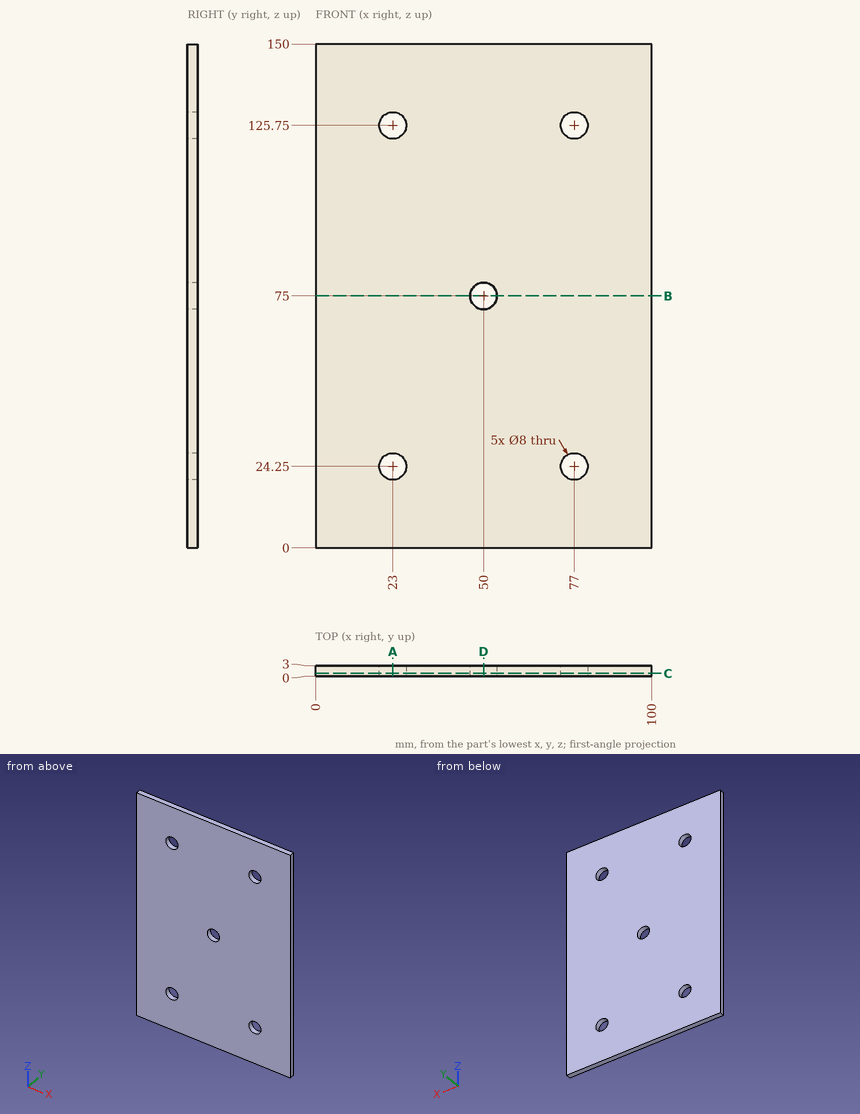
Answer from the drawing. Dimensions are ordinates in mm from the lowest x, y and z of the part. Coordinates: 2 decimals unless noted, no trailing zeros. Loops run counter-clockwise (first coordinate to the right, second up) from the corner with the lowest first, then second, coordinate; pieces in that order, holes last. Notation, with made-up numbers: (48, -34.75) -> (81, -34.75) arc R26 ccw to (81, -1.75) -> close; hole circle Ø6 at (23, -0.5). An arc over 180 degrees is marked (long way). Return JSON: item names as keys, results as strings.
Item 1: Find section D-D (x = 50). Determine the outline of the cut face in (y, z).
Answers:
{"outline": "(0, 0) -> (3, 0) -> (3, 71) -> (0, 71) -> close; (0, 79) -> (3, 79) -> (3, 150) -> (0, 150) -> close"}
Item 2: Find section A-A (x = 23). Determine the outline of the cut face in (y, z).
Answers:
{"outline": "(0, 0) -> (3, 0) -> (3, 20.25) -> (0, 20.25) -> close; (0, 28.25) -> (3, 28.25) -> (3, 121.75) -> (0, 121.75) -> close; (0, 129.75) -> (3, 129.75) -> (3, 150) -> (0, 150) -> close"}
Item 3: Find the intervals of material crossed by probe 1 along Z at (x, y) = (77, 1.8); probe 2 along X at (y, z) = (1.35, 126); probe 3 along X at (y, z) = (1.4, 21.5), in increasing order.
Answers:
{"probe 1": "z = 0 to 20.25, 28.25 to 121.75, 129.75 to 150", "probe 2": "x = 0 to 19.01, 26.99 to 73.01, 80.99 to 100", "probe 3": "x = 0 to 20.1, 25.9 to 74.1, 79.9 to 100"}
Item 4: Find section B-B (z = 75). Determine the outline of the cut face in (x, y).
Answers:
{"outline": "(0, 0) -> (46, 0) -> (46, 3) -> (0, 3) -> close; (54, 0) -> (100, 0) -> (100, 3) -> (54, 3) -> close"}
Item 5: Find section C-C (y = 0.8). Determine the outline of the cut face in (x, z), plus the area to 3 significant figures.
Answers:
{"outline": "(0, 0) -> (100, 0) -> (100, 150) -> (0, 150) -> close; hole circle Ø8 at (23, 24.25); hole circle Ø8 at (23, 125.75); hole circle Ø8 at (50, 75); hole circle Ø8 at (77, 24.25); hole circle Ø8 at (77, 125.75)", "area": "14,700 mm2"}
